from build123d import *

# Parameters (mm, degrees)
CHAMFER1_SIZE      = 0.5
CHAMFER2_SIZE      = 0.3
CUT_EXTRUDE1_DEPTH = 2.5
CHAMFER3_SIZE      = 0.3


with BuildPart() as part:
    # Sketch1 → Revolve1 (revolve)
    with BuildSketch(Plane.XY):
        Polygon((0, 0), (0, 2.75), (3, 2.75), (3, 1.49), (28, 1.49), (28, 0), align=None)
    revolve(axis=Axis((-88.705490849, 0, 0), (1, 0, 0)))

    # Chamfer1
    chamfer1_edges = [part.edges().sort_by_distance(p)[0] for p in [
        (28, -1.49, 0),
    ]]
    chamfer(chamfer1_edges, length=CHAMFER1_SIZE)

    # Chamfer2
    chamfer2_edges = [part.edges().sort_by_distance(p)[0] for p in [
        (0, -2.75, 0),
    ]]
    chamfer(chamfer2_edges, length=CHAMFER2_SIZE)

    # Sketch3 → Cut-Extrude1 (cut)
    with BuildSketch(Plane(origin=(0, 0, 0), x_dir=(0, 0, -1), z_dir=(1, 0, 0))):
        Polygon((-1.443375673, 0), (-0.721687836, -1.25), (0.721687836, -1.25), (1.443375673, 0), (0.721687836, 1.25), (-0.721687836, 1.25), align=None)
    extrude(amount=CUT_EXTRUDE1_DEPTH, mode=Mode.SUBTRACT)

    # Chamfer3
    chamfer3_edges = [part.edges().sort_by_distance(p)[0] for p in [
        (0, 0.625, 1.082531755),
        (0, -0.625, 1.082531755),
        (0, -1.25, 0),
        (0, -0.625, -1.082531755),
        (0, 0.625, -1.082531755),
        (0, 1.25, 0),
    ]]
    chamfer(chamfer3_edges, length=CHAMFER3_SIZE)


solid = part.part
Source: CAD feature listing. Evaluate the final solid. Frame: model axes, mm. A direction names the side the tool comes from. Give positions to 0.01 mm unless a question says otherwise; leave off trailing zeros. Write each loop counter-clockwise with the first axis right and the second up, starting at its lowest first coordinate (ties: lowest second). Pieces come first, ordered by that corner, then holes. Notation, with made-up numbers: M 17,88 L 66,88 A14 ccw 66,110 Z; hole C -38.5,2 d1. An arc over 180 degrees is marked long. Answer as a JSON object with one key per item and string values.
Q1. Cut plane B-B, the plane x = 5. Return the cut outline in (y, z).
Geometry check:
{"outline": "C 0,0 d2.98"}
Q2. Contact query for flat-ended pins moving along their axis: P1, Ø3, axis at y = 0, z = -0.5, coming from the -X side; P2, Ø1, axis at x = 14.5, y = 1, coming from the +Z side; P3, Ø1.5, axis at x = 8, y = 1.5, coming from the +Z side. Output: stop coordinate, or through.
Geometry check:
{"P1": "stops at x = 0", "P2": "stops at z = 1.4", "P3": "stops at z = 1.29"}
Q3. Ray query, line 1 along Y through (x, z) = (24.5, -0.05); line 2 along Z through (x, y) = (1.5, 2.45); line 3 along X through (y, z) = (2.4, -0.35). Return the intervals inside material, ascending.
Geometry check:
{"line 1": "y = -1.49 to 1.49", "line 2": "z = -1.25 to 1.25", "line 3": "x = 0 to 3"}
Q4. Access query for faces 4 (the face through (1.38, 0.63, 1.08)), 5 (the face through (28, 0, 0)). Directions: +Z, -Z, +X, -X, +Y, -Y. A direction counts if a zero-diameter tool reaches every point of the face in a straight line with its end or side. Return the directions, or none.
Geometry check:
{"face 4": "-X", "face 5": "+Z, -Z, +X, +Y, -Y"}
Q5. Mould query, pull axis Y, two halves, no side actions, for faces 1 (the face through (15.422, -0.194, 1.477)), 2 (the face through (3, 1.2, -1.2)), 3 (the face through (1.38, -0.63, -1.08)). Classes: +Y half, -Y half, draft (parallel to the pull), parting line (faces both ways), or undercut.
Geometry check:
{"face 1": "parting line", "face 2": "draft", "face 3": "undercut"}
Q6. Cut plane A-A, the plane z = 0. Return the cut outline in (x, y), then the cut area to 3 significant figures.
Geometry check:
{"outline": "M 0,-2.45 L 0.3,-2.75 L 3,-2.75 L 3,-1.49 L 27.5,-1.49 L 28,-0.99 L 28,0.99 L 27.5,1.49 L 3,1.49 L 3,2.75 L 0.3,2.75 L 0,2.45 L 0,1.55 L 0.3,1.25 L 2.5,1.25 L 2.5,-1.25 L 0.3,-1.25 L 0,-1.55 Z", "area": "84.3 mm^2"}
